Geometry: final body of the model. Coordinates: model frame, mm. Face numbers are marked on the shaded views. Give positions to 0.01 mm unless a question says otherwise; leave off trailing zeros. Write each loop counter-clockwise with the first axis right and the second up, starting at its lowest first coordinate (ties: lowest second). Pieces come first, ordered by that corner, then holes. Notation, with made-up numbers: M 30,10.5 L 78,10.5 A28 ccw 78,37.5 Z; hole C 52,-33.75 d2. An arc over 180 degrees is marked long. Use one line per item in the form item = value. Start each with the question number.
Item 1: Section query B-B on x = -72.5. Return loops of the section in (y, z), then the cut area to 3 significant figures.
Item 2: Section query A-A on z = 1.5. Give the number of separate pieces and of enclosed holes in the cut face, then the cut area to 3 significant figures.
Item 3: Material intervals for line 1 along Y through (x, z) = (87.5, -4.25); line 2 along X through (y, z) = (13, -0.5); line 3 along Y through (x, z) = (-87.5, -3.25), sorted ascending. Write a range as from..to.
Item 4: Pull-direction query (X, two-part tool) for the marked faces 1, 2 and 3; classes: released by +X, released by -X, zero draft, split by the parting line, or undercut.
Item 5: Contact query for flat-ended pins moving along their axis: P1, Ø0.9, axis at x = -86, z = 0.5, coming from the +Y side; P2, Ø0.8, axis at y = 1, z = -3.5, coming from the +X side; P3, Ø5.5, axis at x = 89, y = -13.5, coming from the +Z side. Output: stop coordinate, or through.
from build123d import *

# Parameters (mm, degrees)
SKETCH_2_W                  = 182
SKETCH_2_H                  = 33.5
EXTRUDE_1_DEPTH             = 1.6
SKETCH_3_W                  = 161.4
SKETCH_3_H                  = 28.9
EXTRUDE_2_DEPTH             = 9
SKETCH_4_W                  = 154.4
SKETCH_4_H                  = 16.5
CUT_EXTRUDE_1_DEPTH         = 1
SKETCH_6_R                  = 3.55
EXTRUDE_3_DEPTH             = 5
CUT_EXTRUDE_2_DEPTH         = 94.023343844
CUT_EXTRUDE_2_DEPTH_BACK    = 94.023343844
SKETCH_5_R                  = 1.75
SKETCH_9_W                  = 5
SKETCH_9_H                  = 20.32
EXTRUDE_5_DEPTH             = 2.5
SKETCH_10_W                 = 0.8
SKETCH_10_H                 = 0.8
EXTRUDE_6_DEPTH             = 7
PATTERN_LINEAR_1_COUNT      = 2
PATTERN_LINEAR_1_PITCH      = 2.54
PATTERN_LINEAR_1_COUNT_DIR2 = 8
PATTERN_LINEAR_1_PITCH_DIR2 = 2.54


with BuildPart() as part:
    # Эскиз2 → Бобышка-Вытянуть1 (new body)
    with BuildSketch(Plane.XY.offset(-6.6)):
        Rectangle(SKETCH_2_W, SKETCH_2_H)
    extrude(amount=EXTRUDE_1_DEPTH)

    # Эскиз3 → Бобышка-Вытянуть2 (add)
    with BuildSketch(Plane.XY.offset(-5)):
        with Locations((2.5, 0)):
            Rectangle(SKETCH_3_W, SKETCH_3_H)
    extrude(amount=EXTRUDE_2_DEPTH)

    # Эскиз4 → Вырез-Вытянуть1 (cut)
    with BuildSketch(Plane.XY.offset(4)):
        with Locations((2.5, 0)):
            Rectangle(SKETCH_4_W, SKETCH_4_H)
    extrude(amount=-CUT_EXTRUDE_1_DEPTH, mode=Mode.SUBTRACT)

    # Эскиз6 → Бобышка-Вытянуть3 (add)
    with BuildSketch(Plane(origin=(0, 0, -5), x_dir=(-1, 0, 0), z_dir=(0, 0, -1))):
        with Locations((-87.5, -13.25)):
            Circle(SKETCH_6_R)
        with Locations((-87.5, 13.25)):
            Circle(SKETCH_6_R)
        with Locations((87.5, 13.25)):
            Circle(SKETCH_6_R)
        with Locations((87.5, -13.25)):
            Circle(SKETCH_6_R)
    extrude(amount=-EXTRUDE_3_DEPTH)

    # Эскиз5 → Вырез-Вытянуть2 (cut, two sides: drawn at the far end of the back side and taken through both)
    with BuildSketch(Plane.XY.offset(-5).offset(-CUT_EXTRUDE_2_DEPTH_BACK)):
        with Locations((-87.5, 13.25)):
            Circle(SKETCH_5_R)
        with Locations((-87.5, -13.25)):
            Circle(SKETCH_5_R)
        with Locations((87.5, -13.25)):
            Circle(SKETCH_5_R)
        with Locations((87.5, 13.25)):
            Circle(SKETCH_5_R)
    extrude(amount=CUT_EXTRUDE_2_DEPTH + CUT_EXTRUDE_2_DEPTH_BACK, mode=Mode.SUBTRACT)

    # Эскиз9 → Бобышка-Вытянуть5 (add)
    with BuildSketch(Plane.XY.offset(-5)):
        with Locations((-87.23, 0)):
            Rectangle(SKETCH_9_W, SKETCH_9_H)
    extrude(amount=EXTRUDE_5_DEPTH)

    # Эскиз10 → Бобышка-Вытянуть6 (add)
    with BuildSketch(Plane.XY.offset(-2.5)):
        with Locations((-88.5, 8.95)):
            Rectangle(SKETCH_10_W, SKETCH_10_H)
    extrude_6 = extrude(amount=EXTRUDE_6_DEPTH)

    # Линейный массив1: Extrude 6 2 × 8
    with Locations(*[(i * PATTERN_LINEAR_1_PITCH, -j * PATTERN_LINEAR_1_PITCH_DIR2, 0) for i in range(PATTERN_LINEAR_1_COUNT) for j in range(PATTERN_LINEAR_1_COUNT_DIR2) if (i, j) != (0, 0)]):
        add(extrude_6)


solid = part.part
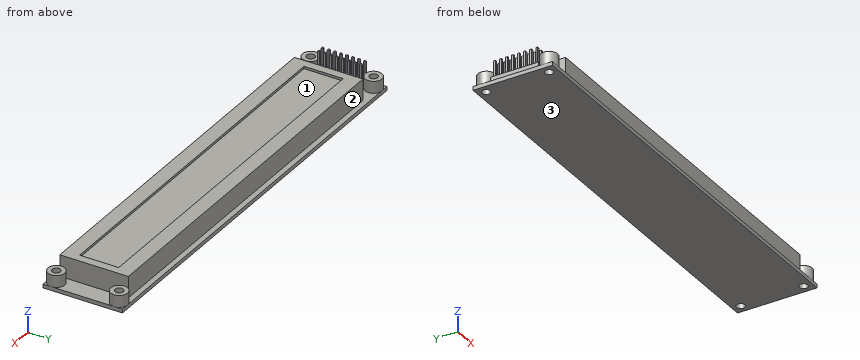
Answer sheet:
q1.outline = M -16.75,-6.6 L 16.75,-6.6 L 16.75,-5 L 14.45,-5 L 14.45,4 L 8.25,4 L 8.25,3 L -8.25,3 L -8.25,4 L -14.45,4 L -14.45,-5 L -16.75,-5 Z
q1.area = 297 mm2
q2.separate_pieces = 17
q2.enclosed_holes = 0
q2.area = 4,670 mm2
q3.line_1 = -16.8..-15, -11.5..-9.7, 9.7..11.5, 15..16.8
q3.line_2 = -91.04..-89.23, -85.77..-83.96, -78.2..83.2, 83.96..85.77, 89.23..91.04
q3.line_3 = -16.8..-15, -11.5..11.5, 15..16.8
q4.face_1 = undercut
q4.face_2 = undercut
q4.face_3 = zero draft
q5.P1 = 9.35
q5.P2 = 83.2
q5.P3 = 0
